Check sheet for the modelled part. Datum: model origin and axes. Units: mm. A direction names the side the tool comes from. Round coordinates to 2 decimals unless told otherwise and drop trailing zeros. Write each loop counter-clockwise with the first axis right and the second up, starting at its lowest first coordinate (ties: lowest second). Pieces come first, ordered by that corner, then holes.
from build123d import *

# Parameters (mm, degrees)
SKETCH1_R           = 31.75
BOSS_EXTRUDE1_DEPTH = 3.175
SKETCH2_R           = 14.2748
BOSS_EXTRUDE2_DEPTH = 36.449
CUT_EXTRUDE1_DEPTH  = 25.4
CUT_EXTRUDE2_DEPTH  = 12.7


with BuildPart() as part:
    # Sketch1 → Boss-Extrude1 (new, symmetric)
    with BuildSketch(Plane.XY):
        Circle(SKETCH1_R)
    extrude(amount=BOSS_EXTRUDE1_DEPTH, both=True)

    # Sketch2 → Boss-Extrude2 (add)
    with BuildSketch(Plane.XY.offset(3.175)):
        Circle(SKETCH2_R)
    extrude(amount=BOSS_EXTRUDE2_DEPTH)

    # Sketch3 → Cut-Extrude1 (cut)
    with BuildSketch(Plane(origin=(0, 0, -3.175), x_dir=(-1, 0, 0), z_dir=(0, 0, -1))):
        with BuildLine():
            Line((-10.066701328, 1.984375), (-10.066701328, -1.984375))
            Line((-10.066701328, -1.984375), (-7.685451328, -1.984375))
            ThreePointArc((-7.685451328, -1.984375), (-6.874076643, -3.96875), (-5.561244824, -5.663608589))
            Line((-5.561244824, -5.663608589), (-6.751869824, -7.725831582))
            Line((-6.751869824, -7.725831582), (-3.314831503, -9.710206582))
            Line((-3.314831503, -9.710206582), (-2.124206503, -7.647983589))
            ThreePointArc((-2.124206503, -7.647983589), (0, -7.9375), (2.124206503, -7.647983589))
            Line((2.124206503, -7.647983589), (3.314831503, -9.710206582))
            Line((3.314831503, -9.710206582), (6.751869824, -7.725831582))
            Line((6.751869824, -7.725831582), (5.561244824, -5.663608589))
            ThreePointArc((5.561244824, -5.663608589), (6.874076643, -3.96875), (7.685451328, -1.984375))
            Line((7.685451328, -1.984375), (10.066701328, -1.984375))
            Line((10.066701328, -1.984375), (10.066701328, 1.984375))
            Line((10.066701328, 1.984375), (7.685451328, 1.984375))
            ThreePointArc((7.685451328, 1.984375), (6.874076643, 3.96875), (5.561244824, 5.663608589))
            Line((5.561244824, 5.663608589), (6.751869824, 7.725831582))
            Line((6.751869824, 7.725831582), (3.314831503, 9.710206582))
            Line((3.314831503, 9.710206582), (2.124206503, 7.647983589))
            ThreePointArc((2.124206503, 7.647983589), (0, 7.9375), (-2.124206503, 7.647983589))
            Line((-2.124206503, 7.647983589), (-3.314831503, 9.710206582))
            Line((-3.314831503, 9.710206582), (-6.751869824, 7.725831582))
            Line((-6.751869824, 7.725831582), (-5.561244824, 5.663608589))
            ThreePointArc((-5.561244824, 5.663608589), (-6.874076643, 3.96875), (-7.685451328, 1.984375))
            Line((-7.685451328, 1.984375), (-10.066701328, 1.984375))
        make_face()
    extrude(amount=-CUT_EXTRUDE1_DEPTH, mode=Mode.SUBTRACT)

    # Sketch4 → Cut-Extrude2 (cut)
    with BuildSketch(Plane.XY.offset(39.624)):
        Polygon((0, 7.332348419), (-6.35, 3.666174209), (-6.35, -3.666174209), (0, -7.332348419), (6.35, -3.666174209), (6.35, 3.666174209), align=None)
    extrude(amount=-CUT_EXTRUDE2_DEPTH, mode=Mode.SUBTRACT)


solid = part.part
1. Sectioned sample at B-B, the plane y = 0. Enter the section's corners in (x, z) (3 decimals).
2. Sectioned sample at D-D, the plane x = -24. Enter the section's corners in (y, z) (3 decimals), plus the area to 3 significant figures.
3. Set-up check for faces 1 (the flat face through (9, 1.984, 9)), 2 (the flat face through (6.35, 0, 33)): record each of +Z, -Z, +X, -X, +Y, -Y from which the full face is reachable in a straight line by a thin tool's end or side.
4. Sectioned sample at C-C, the plane z = 18. Enter the section's corners in (x, y) (1 decimal).
5. Sectioned sample at A-A, the plane z = 31. Enter the section's corners in (x, y), plus the area to 3 significant figures.
6. Scan lines: line 1 along X through (y, z) = (-0.5, 35); line 2 along X through (y, z) = (-8.5, 9); line 3 along Z through (x, y) = (10, 25) (3 decimals). Record each from-to range of solid material in increasing order.
7. Go/stop test with flat-tipped pins: pin 1 (1 mm diameter, centred on x = -25, y = -5, fed in from +Z) (3 decimals); pin 2 (2 mm diameter, centred on x = 3.5, z = 35, fed in from +Y); pin 3 (8 mm diameter, centred on y = -1.5, z = 35, fed in from +X); pin 4 (21.5 mm diameter, centred on x = 3.5, y = 2, fed in from -Z) (3 decimals). Record where each tip stops, or that it passes through.
8. Release check for a two-part mould opening along X. For faces 3 (the cylindrical face through (6.86, 3.99, 9.35)), 4 (the cylindrical face through (-6.883, -30.995, 0.044)) record: released by +X, released by -X, zero draft, split by the parting line, or undercut.
Computed values:
1. outline: (-31.75, -3.175) - (-10.067, -3.175) - (-10.067, 22.225) - (10.067, 22.225) - (10.067, -3.175) - (31.75, -3.175) - (31.75, 3.175) - (14.275, 3.175) - (14.275, 39.624) - (6.35, 39.624) - (6.35, 26.924) - (-6.35, 26.924) - (-6.35, 39.624) - (-14.275, 39.624) - (-14.275, 3.175) - (-31.75, 3.175) - close
2. outline: (-20.786, -3.175) - (20.786, -3.175) - (20.786, 3.175) - (-20.786, 3.175) - close
2. area: 264 mm2
3. face 1: -Z
3. face 2: +Z
4. outline: circle Ø28.5 at (0, 0); hole (-10.1, -2) - (-7.7, -2) arc R7.9 ccw to (-5.6, -5.7) - (-6.8, -7.7) - (-3.3, -9.7) - (-2.1, -7.6) arc R7.9 ccw to (2.1, -7.6) - (3.3, -9.7) - (6.8, -7.7) - (5.6, -5.7) arc R7.9 ccw to (7.7, -2) - (10.1, -2) - (10.1, 2) - (7.7, 2) arc R7.9 ccw to (5.6, 5.7) - (6.8, 7.7) - (3.3, 9.7) - (2.1, 7.6) arc R7.9 ccw to (-2.1, 7.6) - (-3.3, 9.7) - (-6.8, 7.7) - (-5.6, 5.7) arc R7.9 ccw to (-7.7, 2) - (-10.1, 2) - close
5. outline: circle Ø28.55 at (0, 0); hole (-6.35, -3.67) - (0, -7.33) - (6.35, -3.67) - (6.35, 3.67) - (0, 7.33) - (-6.35, 3.67) - close
5. area: 500 mm2
6. line 1: x = -14.27 to -6.35, 6.35 to 14.27
6. line 2: x = -11.47 to -5.41, -2.62 to 2.62, 5.41 to 11.47
6. line 3: z = -3.175 to 3.175
7. pin 1: stops at z = 3.175
7. pin 2: stops at y = 14.05
7. pin 3: stops at x = 14.27
7. pin 4: stops at z = -3.175
8. face 3: undercut
8. face 4: split by the parting line
